Input: part model. Units: mm. Frame: model coordinates. Face numbers are marked on the shaded views. A direction names the side the tool comes from. Give positions to 0.01 mm unless a question says otherwise; leave off trailing zeros. Write each loop counter-clockwise with the first axis right and the second up, starting at its lowest first coordinate (ties: lowest second). Pieces come first, ordered by that corner, then holes. Notation, with made-up numbers: (-29, 52.25) - (25, 52.25) arc R19 cw to (25, 88.25) - close; hole circle Ø10 at (-35, -18). An arc over 180 degrees is marked (long way). Answer as a JSON object with one key per item and string values. Group by question number.
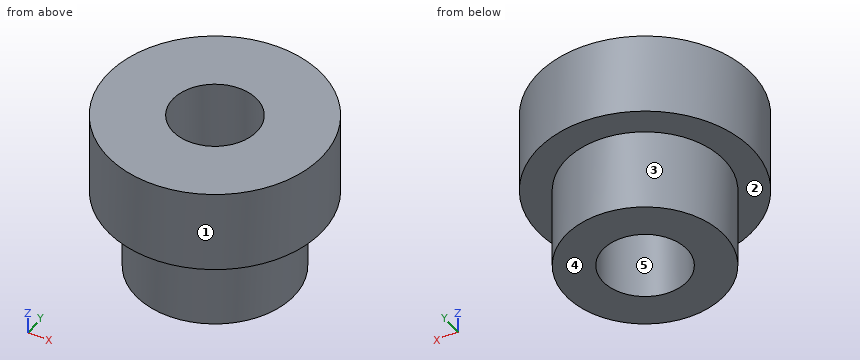
Solid Edge part; units mm, degrees
sketch "Sketch1" plane through (0, 0, 0) normal (0, 0, 1) x (1, 0, 0)
  circle A0 centre (5.1022, 4.5263) radius 6.5
extrude "Protrusion1" add sketch "Sketch1" along normal blind 5
sketch "Sketch2" plane through (5.1022, 4.5263, 0) normal (0, 0, -1) x (-1, 0, 0)
  circle A0 centre (0, 0) radius 4.8
extrude "ExtrudedProtrusion_2" add sketch "Sketch2" along normal blind 5
hole "Hole_1" at (5.1022, 4.5263, -5) direction (0, 0, 1) diameter 5.1 end through all
1) Reachability of the marked faces 1 and 2 from +Z, -Z, +X, -X, +Y, -Y: full face, straight path, thin tool, end or side. Return the list, or none.
2) Line query: line 1 along Z through (x, y) = (10.5, 4.75); line 2 along X through (y, z) = (2.75, -4); line 3 along X through (y, z) = (2.5, -4). Output: solid intervals per line, ascending. Write a range as from..to.
3) Cut plane D-D on z = -3.75. Return the cut outline in (x, y), and give its area (3 significant figures).
4) Cut plane B-B on y = 2.25. Return the cut outline in (x, z).
5) Mould query, pull axis Y, two halves, no side actions, for the marked faces 3, 4 and 5. Classes: +Y half, -Y half, draft (parallel to the pull), parting line (faces both ways), or undercut.
6) Pin query (flat end, axial travel): P1, Ø3, axis at x = 1, y = 1.5, coming from the -Z side; P2, Ø1.5, axis at x = 1.5, z = -4, coming from the -Y side; P3, Ø3, axis at x = 7, z = -2.5, coming from the -Y side; P4, Ø6, axis at y = 1, z = 0.5, coming from the +X side. Return the tip coordinate at first contact, or that it passes through.
7) Cut plane C-C on y = 0.25. Return the cut outline in (x, z).
8) Cut plane A-A on x = 3. Return the cut outline in (y, z).
Filled in:
{
 "1": {"face 1": "+Z, -Z", "face 2": "-Z"},
 "2": {"line 1": "z = 0..5", "line 2": "x = 0.64..3.27, 6.93..9.56", "line 3": "x = 0.75..3.55, 6.65..9.45"},
 "3": {"outline": "circle Ø9.6 at (5.1, 4.53); hole circle Ø5.1 at (5.1, 4.53)", "area": "52.0 mm²"},
 "4": {"outline": "(-0.99, 0) - (0.88, 0) - (0.88, -5) - (3.95, -5) - (3.95, 5) - (-0.99, 5) - close; (6.25, -5) - (9.33, -5) - (9.33, 0) - (11.19, 0) - (11.19, 5) - (6.25, 5) - close"},
 "5": {"face 3": "parting line", "face 4": "draft", "face 5": "undercut"},
 "6": {"P1": "stops at z = -5", "P2": "stops at y = 0.67", "P3": "stops at y = -0.26", "P4": "stops at x = 11.58"},
 "7": {"outline": "(0.21, 0) - (2.92, 0) - (2.92, -5) - (7.28, -5) - (7.28, 0) - (10, 0) - (10, 5) - (0.21, 5) - close"},
 "8": {"outline": "(-1.62, 0) - (0.21, 0) - (0.21, -5) - (3.08, -5) - (3.08, 5) - (-1.62, 5) - close; (5.97, -5) - (8.84, -5) - (8.84, 0) - (10.68, 0) - (10.68, 5) - (5.97, 5) - close"}
}
